The listing builds one solid part. Answer for the finished solid, in the listing's coordinates (mm). A direction names the side the tool comes from. Coordinates: 2 decimals unless noted, no trailing zeros. Order: outer loops, then holes, each group sorted by start corner. A loop starts at its lowest first (then second) coordinate and runs counter-clockwise, first axis right, second up. Notation, with made-up numbers: (38.5, 21.5) - (87.5, 21.5) arc R23 cw to (87.5, 45.5) - close; hole circle Ø7 at (85, 63.25). An arc over 180 degrees is marked (long way). Use one line per item in the form item = value. Start each with the question number.
Item 1: Consider line 1 along X through (y, z) = (-0.5, -28.5); line 2 along Z through (x, y) = (-15, 11); line 3 along X through (y, z) = (35, 35.5). Determine where each line is inside the solid, lowest interval first. Write a range as [from, to].
Item 2: Section A-A, the plane x = -8 is taken. Write down the section's boundary in (y, z), and give its area (3 significant figures).
Item 3: A tool of negligible diameter and unlimited length cuts with its end or side. For faces 5 (the flat face through (-30.9, -29.6, 10)), 6 (the cylindrical face through (-28, -39, 52)), 7 (the cylindrical face through (-39, 28, 52)), 8 (the cylindrical face through (28, 39, 52)), from which of +Z, -Z, +X, -X, +Y, -Y can it reach the whole face along a straight path? Write none if from no direction.
Item 4: Section B-B, the plane y = 0 is taken. Write down the section's boundary in (x, z), and give its area (3 significant figures).
Item 5: Section C-C, the plane z = 17.5 is taken. Write down the section's boundary in (x, y).
Item 6: Section D-D, the plane y = 21 is taken. Write down the section's boundary in (x, z), and give its area (3 significant figures).
Item 7: Each of these flat-tipped pins is pushed along its axis until it touches: pin 1 Ø10 at (x, y) = (22.5, -22.5) entering from -Z; pin 2 Ø1.5 at (x, z) = (-32.5, 42.5) entering from +Y; pin 3 Ø2.5 at (y, z) = (-33, 61) entering from -X. Where does it stop, or does it pass through?
Item 8: The mould has two halves that part along Y. Classify faces 1 (the flat face through (35, -35, 10)), 2 (the flat face through (29.6, -30.6, 10)), 3 (the cylindrical face through (35.237, 32.579, 5.07)), 4 (the flat face through (-33, 30, 53)): released by +Y, released by -Y, zero draft, split by the parting line, or undercut.
from build123d import *

# Parameters (mm, degrees)
SKETCH_1_W          = 80
SKETCH_1_H          = 80
EXTRUDE_1_DEPTH     = 95
SKETCH_2_R          = 10
EXTRUDE_2_DEPTH     = 50
SKETCH_3_W          = 10
SKETCH_3_H          = 10
CUT_EXTRUDE_1_DEPTH = 85
FILLET_1_R          = 10
FILLET_3_R          = 5
MM_1_AT_2_COUNT     = 2
MM_1_AT_2_PITCH     = 63.639610307
MM_1_AT_3_COUNT     = 2
MM_1_AT_3_PITCH     = 90
MM_1_AT_4_COUNT     = 2
MM_1_AT_4_PITCH     = 63.639610307


with BuildPart() as part:
    # 草图1 → 凸台-拉伸1 (new body)
    with BuildSketch(Plane.XY):
        Rectangle(SKETCH_1_W, SKETCH_1_H)
    extrude(amount=EXTRUDE_1_DEPTH)

    # 草图2 → 凸台-拉伸2 (add)
    with BuildSketch(Plane(origin=(0, 0, 0), x_dir=(-1, 0, 0), z_dir=(0, 0, -1))):
        Circle(SKETCH_2_R)
    extrude(amount=EXTRUDE_2_DEPTH)

    # 草图3 → 切除-拉伸1 (cut)
    with BuildSketch(Plane.XY.offset(95)):
        with Locations((-35, 35)):
            Rectangle(SKETCH_3_W, SKETCH_3_H)
        with Locations((35, 35)):
            Rectangle(SKETCH_3_W, SKETCH_3_H)
        with Locations((35, -35)):
            Rectangle(SKETCH_3_W, SKETCH_3_H)
        with Locations((-35, -35)):
            Rectangle(SKETCH_3_W, SKETCH_3_H)
    extrude(amount=-CUT_EXTRUDE_1_DEPTH, mode=Mode.SUBTRACT)

    # 圆角1
    fillet_1_edges = [part.edges().sort_by_distance(p)[0] for p in [
        (40, 40, 5),
        (40, -40, 5),
        (-40, 40, 5),
        (-40, -40, 5),
    ]]
    fillet(fillet_1_edges, radius=FILLET_1_R)

    # 圆角3
    fillet_3_edges = [part.edges().sort_by_distance(p)[0] for p in [
        (-30, -40, 52.5),
        (-40, -30, 52.5),
        (40, -30, 52.5),
        (30, -40, 52.5),
        (30, 40, 52.5),
        (40, 30, 52.5),
        (-40, 30, 52.5),
        (-30, 40, 52.5),
    ]]
    fillet(fillet_3_edges, radius=FILLET_3_R)

    # 草图5 → 大小mm 暗销槽口1 (revolve, cut)
    with BuildSketch(Plane(origin=(-31.819805153, 31.819805153, 10), x_dir=(0, -1, 0), z_dir=(1, 0, 0))):
        Polygon((0, 0), (0, 62.103012167), (3.5, 60), (3.5, 0), align=None)
    mm_1 = revolve(axis=Axis((-31.819805153, 31.819805153, 16.35), (0, 0, -1)), mode=Mode.SUBTRACT)

    # 大小mm 暗销槽口1 at 2: 大小mm 暗销槽口1 ×2
    with Locations(*[(i * MM_1_AT_2_PITCH, 0, 0) for i in range(1, MM_1_AT_2_COUNT)]):
        add(mm_1, mode=Mode.SUBTRACT)

    # 大小mm 暗销槽口1 at 3: 大小mm 暗销槽口1 ×2
    with Locations(*[Vector(0.707106781, -0.707106781, 0) * (i * MM_1_AT_3_PITCH) for i in range(1, MM_1_AT_3_COUNT)]):
        add(mm_1, mode=Mode.SUBTRACT)

    # 大小mm 暗销槽口1 at 4: 大小mm 暗销槽口1 ×2
    with Locations(*[(0, -i * MM_1_AT_4_PITCH, 0) for i in range(1, MM_1_AT_4_COUNT)]):
        add(mm_1, mode=Mode.SUBTRACT)


solid = part.part
Response:
q1.line_1 = [-9.99, 9.99]
q1.line_2 = [0, 95]
q1.line_3 = [-30, 30]
q2.outline = (-40, 0) - (-6, 0) - (-6, -50) - (6, -50) - (6, 0) - (40, 0) - (40, 95) - (-40, 95) - close
q2.area = 8,200 mm2
q3.face_5 = -Z
q3.face_6 = +Z, -X, -Y
q3.face_7 = +Z, -X, +Y
q3.face_8 = +Z, +X, +Y
q4.outline = (-40, 0) - (-10, 0) - (-10, -50) - (10, -50) - (10, 0) - (40, 0) - (40, 95) - (-40, 95) - close
q4.area = 8,600 mm2
q5.outline = (-40, -25) arc R5 ccw to (-35, -30) - (-30, -30) - (-30, -35) arc R5 ccw to (-25, -40) - (25, -40) arc R5 ccw to (30, -35) - (30, -30) - (35, -30) arc R5 ccw to (40, -25) - (40, 25) arc R5 ccw to (35, 30) - (30, 30) - (30, 35) arc R5 ccw to (25, 40) - (-25, 40) arc R5 ccw to (-30, 35) - (-30, 30) - (-35, 30) arc R5 ccw to (-40, 25) - close
q6.outline = (-40, 0) - (40, 0) - (40, 95) - (-40, 95) - close
q6.area = 7,600 mm2
q7.pin_1 = 0
q7.pin_2 = 30
q7.pin_3 = -30
q8.face_1 = zero draft
q8.face_2 = undercut
q8.face_3 = undercut
q8.face_4 = released by +Y
